The model under review builds one solid part; all positions refer to its coordinate system, in mm. A direction names the side the tool comes from. Round coordinates to 2 decimals unless told otherwise and drop trailing zeros.
1) To check wall thickness, follow L1, parallel to Y at x = 0.5, z = -0.5; L2, parallel to Y at x = -3, z = 1; L3, parallel to X at y = 0.75, z = 1.75. State the ranges of each line that lie inside material, in increasing order.
2) Machinability: for faces 1 (the face through (-3.2, 5.66, 0.83)), 2 (the face through (3.3, 5.6, 0.8)), 3 (the face through (3.2, -5.66, 0.83)), 4 (the face through (-3.3, -5.6, 0.8)), which of the approach directions +Z, -Z, +X, -X, +Y, -Y give a long, thin tool a straight path to every point of the face, cutting with its end or side? Answer none if there is none.
3) Clearance check with flat-ended pins moving along their axes: P1, Ø3, axis at y = -1, z = 2, coming from the -X side; P2, Ø3, axis at x = -5.5, z = -2.5, coming from the -Y side; P3, Ø2, axis at y = -2.5, z = -2, coming from the -X side. State where each tip first meets the part, or that it passes through.
from build123d import *

# Parameters (mm, degrees)
EXTRUDE1_DEPTH      = 4
SKETCH2_OUTSIDE_W   = 80.544
SKETCH2_OUTSIDE_H   = 80.544
SKETCH2_OUTSIDE_R   = 6.5
CUT_EXTRUDE1_DEPTH  = 15.97347655
CUT_EXTRUDE1_DRAFT  = -60
SKETCH5_R           = 4
CUT_EXTRUDE10_DEPTH = 15.97347655
SKETCH16_R          = 6.5
SKETCH16_RX         = 4
SKETCH16_RY         = 3.594050592
EXTRUDE2_DEPTH      = 8


with BuildPart() as part:
    # Sketch1 → Extrude1 (new, symmetric)
    with BuildSketch(Plane.XY):
        Polygon((6.5, -3.75277675), (6.5, 3.75277675), (0, 7.505553499), (-6.5, 3.75277675), (-6.5, -3.75277675), (0, -7.505553499), align=None)
    extrude(amount=EXTRUDE1_DEPTH, both=True)

    # Sketch18 → Revolve1 (revolve)
    with BuildSketch(Plane(origin=(0, 0, 0), x_dir=(0, 0, -1), z_dir=(1, 0, 0))):
        with BuildLine():
            Line((4, 0), (4, 8.95))
            Line((4, 8.95), (2.8, 8.95))
            ThreePointArc((2.8, 8.95), (1.901336288, 4.515044297), (1.6, 0))
            Line((1.6, 0), (4, 0))
        make_face()
    revolve(axis=Axis((0, 0, -4), (0, 0, 1)))


with BuildPart() as cut_extrude1_tool:
    # Sketch2 outside → Cut-Extrude1 (with draft: the straight prism first)
    with BuildSketch(Plane.XY.offset(4)):
        Rectangle(SKETCH2_OUTSIDE_W, SKETCH2_OUTSIDE_H)
        Circle(SKETCH2_OUTSIDE_R, mode=Mode.SUBTRACT)
    extrude(amount=-CUT_EXTRUDE1_DEPTH)
    # Cut-Extrude1: the draft: its side faces are tilted about the plane it starts from
    cut_extrude1_sides = [cut_extrude1_tool.faces().sort_by_distance(p)[0] for p in [
        (0, -40.272, -3.986738275),
        (40.272, 0, -3.986738275),
        (0, 40.272, -3.986738275),
        (-40.272, 0, -3.986738275),
        (-6.5, 0, -3.986738275),
    ]]
    draft(cut_extrude1_sides, Plane.XY.offset(4), CUT_EXTRUDE1_DRAFT)


with BuildPart() as part_1:
    add(part.part)

    # Cut-Extrude1: cut by cut_extrude1_tool
    add(cut_extrude1_tool.part, mode=Mode.SUBTRACT)

    # Sketch5 → Cut-Extrude10 (cut, through all)
    with BuildSketch(Plane(origin=(0, 0, 4), x_dir=(-1, 0, 0), z_dir=(0, 0, -1))):
        Circle(SKETCH5_R)
    extrude(amount=CUT_EXTRUDE10_DEPTH, mode=Mode.SUBTRACT)

    # Sketch16 → Extrude2 (add)
    with BuildSketch(Plane.XY.offset(4)):
        Circle(SKETCH16_R)
        with Locations(Location((0, 0), (0, 0, 90))):
            Ellipse(SKETCH16_RX, SKETCH16_RY, mode=Mode.SUBTRACT)
    extrude(amount=-EXTRUDE2_DEPTH)


solid = part_1.part
Answer below:
1. L1: y = -7.22 to -3.96, 3.96 to 7.22
1. L2: y = -5.77 to -2.2, 2.2 to 5.77
1. L3: x = -6.5 to -3.53, 3.53 to 6.5
2. face 1: +Z, -X, +Y
2. face 2: +Z, +X, +Y
2. face 3: +Z, +X, -Y
2. face 4: +Z, -X, -Y
3. P1: stops at x = -6.5
3. P2: stops at y = -7.99
3. P3: stops at x = -8.75
